Can you work these out from the model? Positions are in its coordinate system, mm. Face numbers are marked on the shaded views. A direction names the side the tool comes from. Give positions to 0.01 mm unless a question says otherwise; leave off trailing zeros. Loops run counter-clockwise (first coordinate to the right, second up) from the corner with the lowest first, then second, coordinate; pieces in that order, holes last. Notation, with made-up numbers: (16.5, 50.5) -> (57.5, 50.5) arc R26 ccw to (57.5, 77.5) -> close; hole circle Ø9 at (83, 70.5). An arc over 180 degrees is marked (long way). One line per question, with ' | ' between items.
from build123d import *

# Parameters (mm, degrees)
SKETCH1_W                                    = 46
SKETCH1_H                                    = 46
BOSS_EXTRUDE1_DEPTH                          = 65
SKETCH3_W                                    = 75
SKETCH3_H                                    = 75
SKETCH3_W_2                                  = 52
SKETCH3_H_2                                  = 52
SKETCH3_W_3                                  = 23
SKETCH3_H_3                                  = 46
BOSS_EXTRUDE2_DEPTH                          = 5
SKETCH8_W                                    = 75
SKETCH8_H                                    = 75
SKETCH8_W_2                                  = 52
SKETCH8_H_2                                  = 52
BOSS_EXTRUDE3_DEPTH                          = 5.047079132
FILLET1_R                                    = 2
CBORE_FOR_M6_HEX_SOCKET_HEAD_CAP_SCR_2_COUNT = 2
CBORE_FOR_M6_HEX_SOCKET_HEAD_CAP_SCR_2_PITCH = 50
CBORE_FOR_M6_HEX_SOCKET_HEAD_CAP_SCR_3_COUNT = 2
CBORE_FOR_M6_HEX_SOCKET_HEAD_CAP_SCR_3_PITCH = 63.5
CBORE_FOR_M6_HEX_SOCKET_HEAD_CAP_SCR_4_COUNT = 2
CBORE_FOR_M6_HEX_SOCKET_HEAD_CAP_SCR_4_PITCH = 80.822336022


with BuildPart() as part:
    # Sketch1 → Boss-Extrude1 (new body)
    with BuildSketch(Plane(origin=(0, 0, 0), x_dir=(0, 1, 0), z_dir=(0, 0, 1))):
        Polygon((-26.156583063, 30.146094376), (-29.048003873, 30.146094376), (-29.048003873, -21.853905624), (22.951996127, -21.853905624), (22.951996127, 30.146094376), (15.339697873, 30.146094376), align=None)
        with Locations((-3.048003873, 4.146094376)):
            Rectangle(SKETCH1_W, SKETCH1_H, mode=Mode.SUBTRACT)
    extrude(amount=BOSS_EXTRUDE1_DEPTH)

    # Sketch3 → Boss-Extrude2 (add)
    # profile 1 of 5: a face of its own
    with BuildSketch(Plane(origin=(0, 0, 0), x_dir=(1, 0, 0), z_dir=(0, 0, -1))):
        with Locations((-4.146094376, 3.048003873)):
            Rectangle(SKETCH3_W, SKETCH3_H)
        with Locations((-4.146094376, 3.048003873)):
            Rectangle(SKETCH3_W_2, SKETCH3_H_2, mode=Mode.SUBTRACT)
    # profile 2 of 5: a face of its own
    with BuildSketch(Plane(origin=(0, 0, 0), x_dir=(1, 0, 0), z_dir=(0, 0, -1))):
        Polygon((21.853905624, 29.048003873), (-4.146094376, 29.048003873), (-4.146094376, 26.048003873), (18.853905624, 26.048003873), (18.853905624, -19.951996127), (-4.146094376, -19.951996127), (-4.146094376, -22.951996127), (21.853905624, -22.951996127), align=None)
    # profile 3 of 5: a face of its own
    with BuildSketch(Plane(origin=(0, 0, 0), x_dir=(1, 0, 0), z_dir=(0, 0, -1))):
        Polygon((-4.146094376, 26.048003873), (-4.146094376, 29.048003873), (-30.146094376, 29.048003873), (-30.146094376, -22.951996127), (-4.146094376, -22.951996127), (-4.146094376, -19.951996127), (-27.146094376, -19.951996127), (-27.146094376, 26.048003873), align=None)
    # profile 4 of 5: a face of its own
    with BuildSketch(Plane(origin=(0, 0, 0), x_dir=(1, 0, 0), z_dir=(0, 0, -1))):
        with Locations((7.353905624, 3.048003873)):
            Rectangle(SKETCH3_W_3, SKETCH3_H_3)
    # profile 5 of 5: a face of its own
    with BuildSketch(Plane(origin=(0, 0, 0), x_dir=(1, 0, 0), z_dir=(0, 0, -1))):
        with Locations((-15.646094376, 3.048003873)):
            Rectangle(SKETCH3_W_3, SKETCH3_H_3)
    extrude(amount=BOSS_EXTRUDE2_DEPTH)

    # Sketch8 → Boss-Extrude3 (add)
    with BuildSketch(Plane.XY):
        with Locations((-4.146094376, -3.048003873)):
            Rectangle(SKETCH8_W, SKETCH8_H)
        with Locations((-4.146094376, -3.048003873)):
            Rectangle(SKETCH8_W_2, SKETCH8_H_2, mode=Mode.SUBTRACT)
    extrude(amount=BOSS_EXTRUDE3_DEPTH)

    # Fillet1
    fillet1_edges = [part.edges().sort_by_distance(p)[0] for p in [
        (21.853905624, 22.951996127, 35.023539566),
        (21.853905624, -29.048003873, 35.023539566),
        (-30.146094376, -29.048003873, 35.023539566),
        (-30.146094376, 22.951996127, 35.023539566),
        (-41.646094376, -40.548003873, 0.023539566),
        (33.353905624, -40.548003873, 0.023539566),
        (33.353905624, 34.451996127, 0.023539566),
        (-41.646094376, 34.451996127, 0.023539566),
    ]]
    fillet(fillet1_edges, radius=FILLET1_R)

    # Sketch15 → CBORE for M6 Hex Socket Head Cap Screw2 (revolve, cut)
    with BuildSketch(Plane(origin=(-35.896094376, 21.951996127, 5.047079132), x_dir=(0, -1, 0), z_dir=(1, 0, 0))):
        Polygon((0, 0), (0, 10.047079132), (3.3, 10.047079132), (3.3, 6.4), (5.5, 6.4), (5.5, 0.025), (5.525, 0), align=None)
    cbore_for_m6_hex_socket_head_cap_screw2 = revolve(axis=Axis((-35.896094376, 21.951996127, 11.397079132), (0, 0, -1)), mode=Mode.SUBTRACT)

    # CBORE for M6 Hex Socket Head Cap Scr 2: CBORE for M6 Hex Socket Head Cap Screw2 ×2
    with Locations(*[(0, -i * CBORE_FOR_M6_HEX_SOCKET_HEAD_CAP_SCR_2_PITCH, 0) for i in range(1, CBORE_FOR_M6_HEX_SOCKET_HEAD_CAP_SCR_2_COUNT)]):
        add(cbore_for_m6_hex_socket_head_cap_screw2, mode=Mode.SUBTRACT)

    # CBORE for M6 Hex Socket Head Cap Scr 3: CBORE for M6 Hex Socket Head Cap Screw2 ×2
    with Locations(*[(i * CBORE_FOR_M6_HEX_SOCKET_HEAD_CAP_SCR_3_PITCH, 0, 0) for i in range(1, CBORE_FOR_M6_HEX_SOCKET_HEAD_CAP_SCR_3_COUNT)]):
        add(cbore_for_m6_hex_socket_head_cap_screw2, mode=Mode.SUBTRACT)

    # CBORE for M6 Hex Socket Head Cap Scr 4: CBORE for M6 Hex Socket Head Cap Screw2 ×2
    with Locations(*[Vector(0.7856739006278309, -0.6186408666360874, 0) * (i * CBORE_FOR_M6_HEX_SOCKET_HEAD_CAP_SCR_4_PITCH) for i in range(1, CBORE_FOR_M6_HEX_SOCKET_HEAD_CAP_SCR_4_COUNT)]):
        add(cbore_for_m6_hex_socket_head_cap_screw2, mode=Mode.SUBTRACT)


solid = part.part
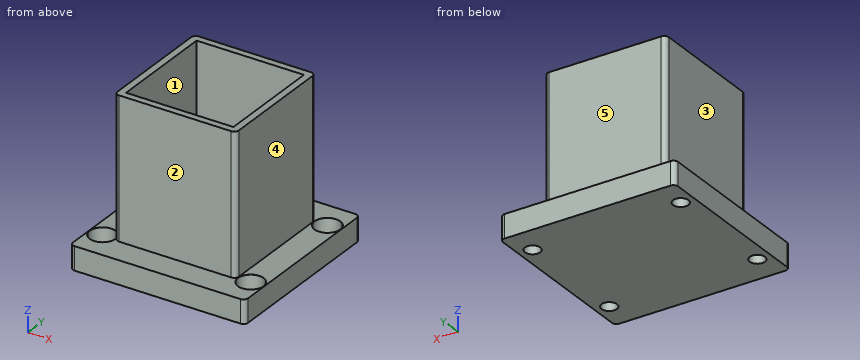
Q1. If we section it at D-D (y = 24): State how many separate pieces and enclosed holes the cut face has, plus the area to 3 significant figures.
Entries:
separate pieces: 3 | enclosed holes: 0 | area: 585 mm²
Q2. If we section it at B-B (x = -17.5): Write out the boundary of the cut face in (y, z).
Entries:
outline: (-40.55, -5) -> (34.45, -5) -> (34.45, 5.05) -> (22.95, 5.05) -> (22.95, 65) -> (19.95, 65) -> (19.95, 0) -> (-26.05, 0) -> (-26.05, 65) -> (-29.05, 65) -> (-29.05, 5.05) -> (-40.55, 5.05) -> close
Q3. If we section it at C-C (y = -10): Write out the boundary of the cut face in (x, z).
Entries:
outline: (-41.65, -5) -> (33.35, -5) -> (33.35, 5.05) -> (21.85, 5.05) -> (21.85, 65) -> (18.85, 65) -> (18.85, 0) -> (-27.15, 0) -> (-27.15, 65) -> (-30.15, 65) -> (-30.15, 5.05) -> (-41.65, 5.05) -> close
Q4. On a 3-axis mill with a long thin cutter (end or side, diameter ignored), from which of +Z, -Z, +X, -X, +Y, -Y can I reach the whole of each face in a straight line? I mean the marked faces 1, 2, 3, 4 and 5. Say none if no direction works.
Entries:
face 1: +Z | face 2: +Z, +X, -X, -Y | face 3: +Z, -X, +Y, -Y | face 4: +Z, +X, +Y, -Y | face 5: +Z, +X, -X, +Y
Q5. If I drill on probe 1 along X at (y, z) = (16, 52.5); probe 2 along Y at (x, z) = (7.5, 8); probe 3 along Y at (x, z) = (-32, 3), over which ranges is the centre line in solid material (lowest first)? Write a range as from..to.
Entries:
probe 1: -30.15..-27.15, 18.85..21.85 | probe 2: -29.05..-26.05, 19.95..22.95 | probe 3: -40.55..-31.93, -24.17..18.07, 25.83..34.45
Q6. For pin 1 Ø9 at (x, y) = (26.5, 19.5) entering from +Z; pin 2 Ø9 at (x, y) = (-35.9, -28.05) entering from +Z; pin 3 Ø6 at (x, y) = (-35.9, -28.05) entering from +Z; pin 4 Ø23 at (x, z) = (-10, 37) entering from -Y, each with a flat end and sliding along its axis, tell me the tip position at first contact or that it passes through.
Entries:
pin 1: z = 5.05 | pin 2: z = -1.35 | pin 3: through | pin 4: y = -29.05
Q7. If we section it at A-A (z = 17): Write out the boundary of the cut face in (x, y), plus the area to 3 significant figures.
Entries:
outline: (-30.15, -27.05) arc R2 ccw to (-28.15, -29.05) -> (19.85, -29.05) arc R2 ccw to (21.85, -27.05) -> (21.85, 20.95) arc R2 ccw to (19.85, 22.95) -> (-28.15, 22.95) arc R2 ccw to (-30.15, 20.95) -> close; hole (-27.15, -26.05) -> (18.85, -26.05) -> (18.85, 19.95) -> (-27.15, 19.95) -> close | area: 585 mm²
